```python
from build123d import *

# Parameters (mm, degrees)
SKETCH_1_R          = 2.85
EXTRUDE_1_DEPTH     = 1.65
SKETCH_2_R          = 1.5
EXTRUDE_2_DEPTH     = 6.5
FILLET_1_R          = 1
CUT_EXTRUDE_1_DEPTH = 1
CHAMFER_1_SIZE      = 0.2


with BuildPart() as part:
    # 草图1 → 凸台-拉伸1 (new body)
    with BuildSketch(Plane.XY):
        Circle(SKETCH_1_R)
    extrude(amount=EXTRUDE_1_DEPTH)

    # 草图2 → 凸台-拉伸2 (add)
    with BuildSketch(Plane(origin=(0, 0, 0), x_dir=(-1, 0, 0), z_dir=(0, 0, -1))):
        with Locations(Location((0, 0, 0), (0, 0, 180))):
            Circle(SKETCH_2_R)
    extrude(amount=EXTRUDE_2_DEPTH)

    # 圆角1
    fillet_1_edges = [part.edges().sort_by_distance(p)[0] for p in [
        (-2.85, 0, 1.65),
    ]]
    fillet(fillet_1_edges, radius=FILLET_1_R)

    # 草图3 → 切除-拉伸1 (cut)
    with BuildSketch(Plane.XY.offset(1.65)):
        Polygon((0.362222341, -1.09641612), (1.130635384, -0.234514311), (0.768413043, 0.861901809), (-0.362222341, 1.09641612), (-1.130635384, 0.234514311), (-0.768413043, -0.861901809), align=None)
    extrude(amount=-CUT_EXTRUDE_1_DEPTH, mode=Mode.SUBTRACT)

    # 倒角1
    chamfer_1_edges = [part.edges().sort_by_distance(p)[0] for p in [
        (-0.203095351, -0.979158965, 0.65),
        (-0.949524213, -0.313693749, 0.65),
        (-0.746428862, 0.665465216, 0.65),
        (0.203095351, 0.979158965, 0.65),
        (0.949524213, 0.313693749, 0.65),
        (0.746428862, -0.665465216, 0.65),
        (-0.203095351, -0.979158965, 1.65),
        (0.746428862, -0.665465216, 1.65),
        (0.949524213, 0.313693749, 1.65),
        (0.203095351, 0.979158965, 1.65),
        (-0.746428862, 0.665465216, 1.65),
        (-0.949524213, -0.313693749, 1.65),
    ]]
    chamfer(chamfer_1_edges, length=CHAMFER_1_SIZE)


solid = part.part
```
Geometry check sheet. Reference: the model listing, model coordinates, mm. A direction names the side the tool comes from. Round coordinates to 2 decimals unless told otherwise and drop trailing zeros. Order: outer loops, then holes, each group sorted by start corner. A loop starts at its lowest first (then second) coordinate and runs counter-clockwise, first axis right, second up. Notation, with made-up numbers: (62.5, 88.5) -> (74.5, 88.5) arc R8 cw to (74.5, 96.5) -> close; hole circle Ø9 at (22.5, 19.5). An arc over 180 degrees is marked (long way). Return JSON: item names as keys, results as strings. Group by question number.
Q1. Material ranges on probe 1 along Y at (x, z) = (0, 1); probe 2 along Y at (x, z) = (-0.6, 0.75); probe 3 along X at (y, z) = (-0.9, -3.5), recorded low to high. Write a range as from..to.
Q2. Section check B-B, the plane z = -5.5. Record the boundary of the cut face in (x, y), plus the area to 3 significant figures.
Q3. Tool access check on faces 4 (the cylindrical face through (1.43, -0.45, -3.2)), 5 (the flat face through (0.4, 1.3, 1.65)). Record the directions out of +Z, -Z, +X, -X, +Y, -Y that give a thin tool (end or side, any length) a straight path to the whole face; none if there is none.
Q4. Gauge pin test, flat ends, axial feed: pin 1 (3 mm diameter, centred on y = 0, z = -4, fed in from +X); pin 2 (1.4 mm diameter, centred on x = 0, y = 0, fed in from +Z); pin 3 (2 mm diameter, centred on x = -0.5, z = -2.5, fed in from +Y). Record the tip position at first contact, or that the pin passes through.
Q5. Release check for a two-part mould opening along X. For faces 1 (the flat face through (0, 0, 0.65)), 2 (the flat face through (1.2, -1.2, 0)), 3 (the cylindrical face through (-2.262, -1.734, 0.32)) record: released by +X, released by -X, zero draft, split by the parting line, or undercut.
Q6. Section check A-A, the plane x = 0. Record the boundary of the cut face in (y, z), plus the area to 3 significant figures.
Numbers:
{
 "1": {"probe 1": "-2.79..-1.02, 1.02..2.79", "probe 2": "-2.78..-0.79, 0.68..2.78", "probe 3": "-1.2..1.2"},
 "2": {"outline": "circle Ø3 at (0, 0)", "area": "7.07 mm^2"},
 "3": {"face 4": "-Z", "face 5": "+Z, +X, -X, +Y, -Y"},
 "4": {"pin 1": "x = 1.5", "pin 2": "z = 0.65", "pin 3": "y = 1.5"},
 "5": {"face 1": "undercut", "face 2": "zero draft", "face 3": "split by the parting line"},
 "6": {"outline": "(-2.85, 0) -> (-1.5, 0) -> (-1.5, -6.5) -> (1.5, -6.5) -> (1.5, 0) -> (2.85, 0) -> (2.85, 0.65) arc R1 ccw to (1.85, 1.65) -> (1.23, 1.65) -> (1.02, 1.45) -> (1.02, 0.85) -> (0.82, 0.65) -> (-0.82, 0.65) -> (-1.02, 0.85) -> (-1.02, 1.45) -> (-1.23, 1.65) -> (-1.85, 1.65) arc R1 ccw to (-2.85, 0.65) -> close", "area": "26.4 mm^2"}
}
